Design review of the part built by this model. Coordinates are the model's own, in mm. Face numbers are marked on the shaded views. Coordinates: 2 decimals unless noted, no trailing zeros.
Q1. For L1, parallel to Y at x = -10, z = 6.5; L2, parallel to Y at x = 6, z = 10; L3, parallel to Y at x = -5.5, z = -16, list the stretches that pass through material, from the lowest coordinate up.
Q2. Take a section at A-A, the plane x = 0. State how many separate pieces and enclosed holes the cut face has, plus the area to 3 significant figures.
Q3. For pin 1 Ø3.5 at (x, y) = (25.5, -13) entering from -Z; pin 2 Ø9.5 at (x, z) = (-2.5, 5.5) entering from -Y; pin 3 Ø2 at (x, y) = (25, -13) entering from +Z, all flat-tipped, find the tip position at first contact; note any pin that passes through.
Q4. The part is to be moulded in two halves that separate along X. For the marked faces 1, 2, 3 and 4, say which applies: released by +X, released by -X, zero draft, split by the parting line, or undercut.
from build123d import *

# Parameters (mm, degrees)
ESQUISSE2_W             = 1.7125
ESQUISSE2_H             = 1.5
ENL_V_MAT_EXTRU_2_REACH = 59.697
BOSS_EXTRU_2_DEPTH      = 0.5
ESQUISSE5_W             = 1
ESQUISSE5_H             = 4
BOSS_EXTRU_3_DEPTH      = 0.5


with BuildPart() as part:
    # Esquisse1 → Base-Révolution (revolve)
    with BuildSketch(Plane.XY, mode=Mode.PRIVATE) as base_r_volution_sk:
        with BuildLine():
            Line((0, 0), (-16, 0))
            Line((-16, 0), (-16, -8))
            Line((-16, -8), (-10, -8))
            Line((-10, -8), (-10, -9))
            Line((-10, -9), (-18, -9))
            Line((-18, -9), (-18, -11))
            Line((-18, -11), (-36, -16))
            Line((-36, -16), (-36, -19))
            Line((-36, -19), (-38, -19))
            Line((-38, -19), (-38, -21))
            Line((-38, -21), (-32, -21))
            Line((-32, -21), (-32, -19))
            Line((-32, -19), (-30, -19))
            Line((-30, -19), (-30, -21))
            Line((-30, -21), (-10, -16))
            ThreePointArc((-10, -16), (-5.360654987, -18.865907042), (0, -19.866068747))
            Line((0, -19.866068747), (0, 0))
        make_face()
    revolve(base_r_volution_sk.sketch.rotate(Axis((0, 70, 0), (0, -1, 0)), 270), axis=Axis((0, 70, 0), (0, -1, 0)))

    # Esquisse2 → Enlèvement de matière-Révolution1 (revolve, cut)
    with BuildSketch(Plane.XY, mode=Mode.PRIVATE) as enl_vement_de_mati_re_r_volution1_sk:
        Polygon((-33.010953329, -16), (-15.010953329, -11), (-5.3, -11), (-5.3, -11.325), (-32, -18), (-33.010953329, -18), align=None)
        with Locations((-15.14375, -0.75)):
            Rectangle(ESQUISSE2_W, ESQUISSE2_H)
    revolve(enl_vement_de_mati_re_r_volution1_sk.sketch.rotate(Axis((0, 0, 0), (0, -1, 0)), 270), axis=Axis((0, 0, 0), (0, -1, 0)), mode=Mode.SUBTRACT)

    # Esquisse3 → Enlèv. mat.-Extru.2 (cut, up to next)
    with BuildSketch(Plane(origin=(0, 0, 0), x_dir=(1, 0, 0), z_dir=(0, 1, 0)), mode=Mode.PRIVATE) as enl_v_mat_extru_2_sk1:
        with BuildLine():
            Line((6, 19.078784028), (6, 31.432467291))
            ThreePointArc((6, 31.432467291), (22.627416998, 22.627416998), (31.432467291, 6))
            Line((31.432467291, 6), (19.078784028, 6))
            ThreePointArc((19.078784028, 6), (14.142135624, 14.142135624), (6, 19.078784028))
        make_face()
    enl_v_mat_extru_2_tool1 = extrude(enl_v_mat_extru_2_sk1.sketch, amount=-ENL_V_MAT_EXTRU_2_REACH, mode=Mode.PRIVATE) & part.part
    # Esquisse3 → Enlèv. mat.-Extru.2 (cut, up to next)
    with BuildSketch(Plane(origin=(0, 0, 0), x_dir=(1, 0, 0), z_dir=(0, 1, 0)), mode=Mode.PRIVATE) as enl_v_mat_extru_2_sk2:
        with BuildLine():
            Line((-6, 19.078784028), (-6, 31.432467291))
            ThreePointArc((-6, 31.432467291), (-22.627416998, 22.627416998), (-31.432467291, 6))
            Line((-31.432467291, 6), (-19.078784028, 6))
            ThreePointArc((-19.078784028, 6), (-14.142135624, 14.142135624), (-6, 19.078784028))
        make_face()
    enl_v_mat_extru_2_tool2 = extrude(enl_v_mat_extru_2_sk2.sketch, amount=-ENL_V_MAT_EXTRU_2_REACH, mode=Mode.PRIVATE) & part.part
    # Esquisse3 → Enlèv. mat.-Extru.2 (cut, up to next)
    with BuildSketch(Plane(origin=(0, 0, 0), x_dir=(1, 0, 0), z_dir=(0, 1, 0)), mode=Mode.PRIVATE) as enl_v_mat_extru_2_sk3:
        with BuildLine():
            Line((-19.078784028, -6), (-31.432467291, -6))
            ThreePointArc((-31.432467291, -6), (-22.627416998, -22.627416998), (-6, -31.432467291))
            Line((-6, -31.432467291), (-6, -19.078784028))
            ThreePointArc((-6, -19.078784028), (-14.142135624, -14.142135624), (-19.078784028, -6))
        make_face()
    enl_v_mat_extru_2_tool3 = extrude(enl_v_mat_extru_2_sk3.sketch, amount=-ENL_V_MAT_EXTRU_2_REACH, mode=Mode.PRIVATE) & part.part
    # Esquisse3 → Enlèv. mat.-Extru.2 (cut, up to next)
    with BuildSketch(Plane(origin=(0, 0, 0), x_dir=(1, 0, 0), z_dir=(0, 1, 0)), mode=Mode.PRIVATE) as enl_v_mat_extru_2_sk4:
        with BuildLine():
            Line((6, -19.078784028), (6, -31.432467291))
            ThreePointArc((6, -31.432467291), (22.627416998, -22.627416998), (31.432467291, -6))
            Line((31.432467291, -6), (19.078784028, -6))
            ThreePointArc((19.078784028, -6), (14.142135624, -14.142135624), (6, -19.078784028))
        make_face()
    enl_v_mat_extru_2_tool4 = extrude(enl_v_mat_extru_2_sk4.sketch, amount=-ENL_V_MAT_EXTRU_2_REACH, mode=Mode.PRIVATE) & part.part
    add(enl_v_mat_extru_2_tool1.solids().sort_by_distance((17.884719, 0, -17.884719))[0], mode=Mode.SUBTRACT)
    add(enl_v_mat_extru_2_tool2.solids().sort_by_distance((-17.884719, 0, -17.884719))[0], mode=Mode.SUBTRACT)
    add(enl_v_mat_extru_2_tool3.solids().sort_by_distance((-17.884719, 0, 17.884719))[0], mode=Mode.SUBTRACT)
    add(enl_v_mat_extru_2_tool4.solids().sort_by_distance((17.884719, 0, 17.884719))[0], mode=Mode.SUBTRACT)

    # Esquisse4 → Boss.-Extru.2 (add, symmetric)
    with BuildSketch(Plane(origin=(27, -13.5, 0), x_dir=(0, 0, -1), z_dir=(0.26764386378609417, 0.9635179096299408, 0))):
        with BuildLine():
            Line((-9, 3.357510793), (9, 3.357510793))
            ThreePointArc((9, 3.357510793), (9.707106781, 3.064617574), (10, 2.357510793))
            Line((10, 2.357510793), (10, 0.357510793))
            ThreePointArc((10, 0.357510793), (9.707106781, -0.349595989), (9, -0.642489207))
            Line((9, -0.642489207), (-9, -0.642489207))
            ThreePointArc((-9, -0.642489207), (-9.707106781, -0.349595989), (-10, 0.357510793))
            Line((-10, 0.357510793), (-10, 2.357510793))
            ThreePointArc((-10, 2.357510793), (-9.707106781, 3.064617574), (-9, 3.357510793))
        make_face()
    extrude(amount=BOSS_EXTRU_2_DEPTH, both=True)

    # Esquisse5 → Boss.-Extru.3 (add)
    with BuildSketch(Plane(origin=(-1.413456005, -5.088441618, 0), x_dir=(-0.9635179096299408, 0.26764386378609417, 0), z_dir=(0.26764386378609417, 0.9635179096299408, 0))):
        with Locations((-28.270664928, 10)):
            Rectangle(ESQUISSE5_W, ESQUISSE5_H)
        with Locations((-28.270664928, -10)):
            Rectangle(ESQUISSE5_W, ESQUISSE5_H)
    extrude(amount=BOSS_EXTRU_3_DEPTH)


solid = part.part
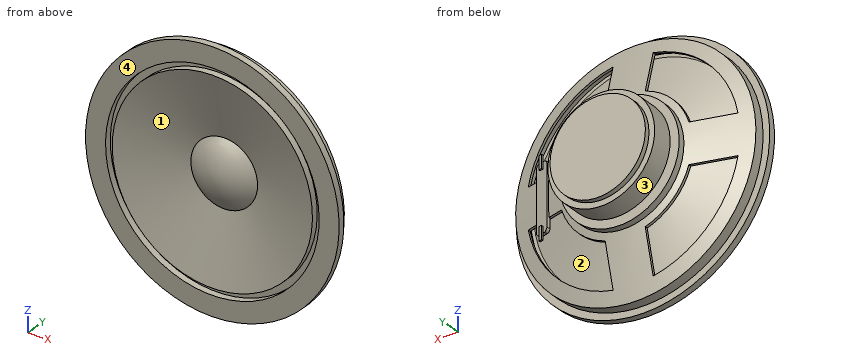
Responses:
1. L1: y = -16.48 to -12.98, -11 to -9, -8 to 0
1. L2: y = -16.42 to -12.92, -11 to -9, -8 to 0
1. L3: y = -17.73 to -14.23, -11.53 to -9
2. separate pieces: 1
2. enclosed holes: 2
2. area: 706 mm2
3. pin 1: stops at z = -12
3. pin 2: stops at y = -19.81
3. pin 3: stops at z = 12
4. face 1: undercut
4. face 2: undercut
4. face 3: split by the parting line
4. face 4: zero draft
